Model file for the job. Use its own axes, mm. A direction names the side the tool comes from. Give positions to 0.01 mm unless a question says otherwise; leave off trailing zeros.
```python
from build123d import *

# Parameters (mm, degrees)
SKETCH1_R           = 50
EXTRUDE1_DEPTH      = 10
EXTRUDE2_DEPTH      = 10
CIRPATTERN1_COUNT   = 16
SKETCH3_R           = 42.5
CUT_EXTRUDE1_DEPTH  = 2
EXTRUDE3_DEPTH      = 10
EXTRUDE3_DEPTH_BACK = 20
SKETCH4_R           = 25
SKETCH4_R_2         = 12.5


with BuildPart() as part:
    # Sketch1 → Extrude1 (new body)
    with BuildSketch(Plane(origin=(-35.411572528, 65.609323585, -43.044793763), x_dir=(0.661608716570187, 0.6269595397180289, -0.4113339783131309), z_dir=(0.411333978313131, -0.7621052147079792, -0.49999999999999767))):
        with Locations(Location((-35.411572528, 65.609323585, 0), (0, 0, 313.459706489))):
            Circle(SKETCH1_R)
    extrude(amount=EXTRUDE1_DEPTH)

    # Sketch2 → Extrude2 (add)
    with BuildSketch(Plane(origin=(-13.592446481, 25.183609646, 16.522396881), x_dir=(0.661608716570187, 0.6269595397180289, -0.4113339783131309), z_dir=(0.4113339783131311, -0.7621052147079793, -0.4999999999999976))):
        Polygon((-3, 60), (3, 60), (8.358983849, 40), (-8.358983849, 40), align=None)
    extrude2 = extrude(amount=-EXTRUDE2_DEPTH)

    # CirPattern1: Extrude2 ×16 about axis
    cirpattern1_axis = Axis((0, 0, 0), (-0.41133397831313073, 0.7621052147079793, 0.4999999999999978))
    for i in range(1, CIRPATTERN1_COUNT):
        add(extrude2.rotate(cirpattern1_axis, i * 360 / CIRPATTERN1_COUNT))

    # Sketch3 → Cut-Extrude1 (cut)
    with BuildSketch(Plane(origin=(-13.592446481, 25.183609646, 16.522396881), x_dir=(0.661608716570187, 0.6269595397180289, -0.4113339783131309), z_dir=(0.4113339783131311, -0.7621052147079793, -0.4999999999999976))):
        with Locations(Location((0, 0, 0), (0, 0, 313.459706489))):
            Circle(SKETCH3_R)
    extrude(amount=-CUT_EXTRUDE1_DEPTH, mode=Mode.SUBTRACT)

    # Sketch4 → Extrude3 (add, two sides: drawn at the far end of the back side and taken through both)
    with BuildSketch(Plane(origin=(-14.415114438, 26.707820075, 17.522396881), x_dir=(0.661608716570187, 0.626959539718029, -0.41133397831313107), z_dir=(0.4113339783131311, -0.7621052147079793, -0.49999999999999756)).offset(-EXTRUDE3_DEPTH_BACK)):
        with Locations(Location((0, 0, 0), (0, 0, 313.459706489))):
            Circle(SKETCH4_R)
        with Locations(Location((0, 0, 0), (0, 0, 313.459706489))):
            Circle(SKETCH4_R_2, mode=Mode.SUBTRACT)
    extrude(amount=EXTRUDE3_DEPTH + EXTRUDE3_DEPTH_BACK)


solid = part.part
```
1. Probe probe 1 along Z at (x, y) = (-22, 26); probe 2 along Z at (x, y) = (-62, -5); probe 3 along X at (y, z) = (62, 2.5). List the from-to ranges inside material, lowest first.
Calculated:
probe 1: z = -7.64 to 7.29, 12.36 to 28.36, 31.19 to 46.95
probe 2: z = 22.71 to 25.43
probe 3: x = 13.26 to 21.2
2. Pull direction Y, two halves, no side cores. Call faces 4 (the flat face through (-70.29, 9.22, 4.07)), 5 (the cylindrical face through (-60.59, 7.44, 15.04)), 6 (the flat face through (1.134, 63.744, -20.277)), 7 (the cylindrical face through (-7.941, 4.937, 62.172)): +Y half, -Y half, draft (parallel to the pull), parting line (faces both ways), or undercut.
Calculated:
face 4: -Y half
face 5: undercut
face 6: +Y half
face 7: undercut
3. Which spindle directions (+Z, -Z, +X, -X, +Y, -Y) get a long thin tool onto all of the face, cutting with end or side? Do faces 1 (the flat face through (32.43, 55.56, 17.94)), 2 (the flat face through (-17.5, 32.8, 21.7)), 3 (the flat face through (15.8, 17.3, 62.5)). Say none if no direction does.
Calculated:
face 1: +X
face 2: none
face 3: +Z, -Y
4. Pin check, flat tips, straight feed: P1, Ø10, axis at y = 57.5, z = 1.5, coming from the -X side; P2, Ø10, axis at x = -18.5, y = 50.5, coming from the +Z side; P3, Ø4, axis at x = -12, y = 8.5, coming from the -Z side. Stop position of each tip, or through.
Calculated:
P1: stops at x = -7.37
P2: stops at z = 23.41
P3: stops at z = 23.8
